Part model, mm, in its own coordinate system. Coordinates: 2 decimals unless noted, no trailing zeros. Order: outer loops, then holes, each group sorted by start corner. A loop starts at its lowest first (then second) coordinate and runs counter-clockwise, first axis right, second up.
from build123d import *

# Parameters (mm, degrees)
CROQUIS1_W              = 1016
CROQUIS1_H              = 76.2
SALIENTE_EXTRUIR1_DEPTH = 50.8
CROQUIS2_R              = 19.05
CORTAR_EXTRUIR1_DEPTH   = 512.953367017
CROQUIS5_R              = 19.05
CORTAR_EXTRUIR3_DEPTH   = 517.188996396
CROQUIS6_W              = 50.8
CROQUIS6_H              = 76.2
SALIENTE_EXTRUIR2_DEPTH = 127
CROQUIS7_R              = 19.05
CORTAR_EXTRUIR4_DEPTH   = 639.167101941


with BuildPart() as part:
    # Croquis1 → Saliente-Extruir1 (new body)
    with BuildSketch(Plane.XY):
        Rectangle(CROQUIS1_W, CROQUIS1_H)
    extrude(amount=SALIENTE_EXTRUIR1_DEPTH)

    # Croquis2 → Cortar-Extruir1 (cut, through all)
    with BuildSketch(Plane.XY.offset(50.8)):
        with Locations((-393.7, 0)):
            Circle(CROQUIS2_R)
    extrude(amount=-CORTAR_EXTRUIR1_DEPTH, mode=Mode.SUBTRACT)

    # Croquis5 → Cortar-Extruir3 (cut, through all)
    with BuildSketch(Plane(origin=(0, 38.1, 0), x_dir=(1, 0, 0), z_dir=(0, 1, 0))):
        with Locations(Location((471.22697118, -25.4, 0), (0, 0, 180))):
            Circle(CROQUIS5_R)
    extrude(amount=-CORTAR_EXTRUIR3_DEPTH, mode=Mode.SUBTRACT)

    # Croquis6 → Saliente-Extruir2 (add)
    with BuildSketch(Plane.ZY.offset(508)):
        with Locations((25.4, 0)):
            Rectangle(CROQUIS6_W, CROQUIS6_H)
    extrude(amount=SALIENTE_EXTRUIR2_DEPTH)

    # Croquis7 → Cortar-Extruir4 (cut, through all)
    with BuildSketch(Plane.XY.offset(50.8)):
        with Locations((-579.845937481, 0)):
            Circle(CROQUIS7_R)
    extrude(amount=-CORTAR_EXTRUIR4_DEPTH, mode=Mode.SUBTRACT)


solid = part.part
Q1. Cut at B-B on x = -393.7. Write the cut outline in (y, z).
Results list:
outline: (-38.1, 0) - (-19.05, 0) - (-19.05, 50.8) - (-38.1, 50.8) - close; (19.05, 0) - (38.1, 0) - (38.1, 50.8) - (19.05, 50.8) - close
Q2. Mould opens along Z. For faces 1 (the face through (462.437, 0.533, 8.499)), 2 (the face through (-55, -1, 50.8)), 3 (the face through (-55, -1, 0)), 4 (the face through (508, -1, 25)) say: pulls with the +Z half, pulls with the -Z half, needs draft (parallel to the pull), parting line crosses it, or undercut.
Results list:
face 1: undercut
face 2: pulls with the +Z half
face 3: pulls with the -Z half
face 4: needs draft
Q3. Wall check: line 1 along X through (y, z) = (1, 25); line 2 along X through (y, z) = (-21, 25); line 3 along X through (y, z) = (4.5, 12). Give the ranges that are in metal, low to high.
Results list:
line 1: x = -635 to -598.87, -560.82 to -412.72, -374.68 to 452.18, 490.27 to 508
line 2: x = -635 to 452.18, 490.27 to 508
line 3: x = -635 to -598.36, -561.34 to -412.21, -375.19 to 457.69, 484.77 to 508
Q4. Cut at A-A on z = 25.4. Write the cut outline in (x, y).
Results list:
outline: (-635, -38.1) - (452.18, -38.1) - (452.18, 38.1) - (-635, 38.1) - close; (490.28, -38.1) - (508, -38.1) - (508, 38.1) - (490.28, 38.1) - close; hole circle Ø38.1 at (-579.85, 0); hole circle Ø38.1 at (-393.7, 0)
